```python
from build123d import *

# Parameters (mm, degrees)
F0_W     = 50.8
F0_H     = 50.8
F1_DEPTH = 6.35
F2_W     = 50.8
F2_H     = 6.35
F3_DEPTH = 6.604
F4_W     = 50.8
F4_H     = 50.8
F5_DEPTH = 6.35
F6_R     = 10.16
F6_R_2   = 8.255
F7_DEPTH = 50.8


with BuildPart() as f1:
    # F0 (on Top) → F1 (new body)
    with BuildSketch(Plane.XY):
        Rectangle(F0_W, F0_H)
    extrude(amount=F1_DEPTH)

    # F2 (on face) → F3 (join)
    with BuildSketch(Plane.XY.offset(6.35)):
        with Locations((0, 22.225)):
            Rectangle(F2_W, F2_H)
    extrude(amount=F3_DEPTH)

    # F4 (on face) → F5 (join)
    with BuildSketch(Plane.XY.offset(12.954)):
        Rectangle(F4_W, F4_H)
    extrude(amount=F5_DEPTH)

    # F6 (on face) → F7 (join)
    with BuildSketch(Plane.XY.offset(19.304)):
        Circle(F6_R)
        Circle(F6_R_2, mode=Mode.SUBTRACT)
    extrude(amount=F7_DEPTH)


solid = f1.part
```
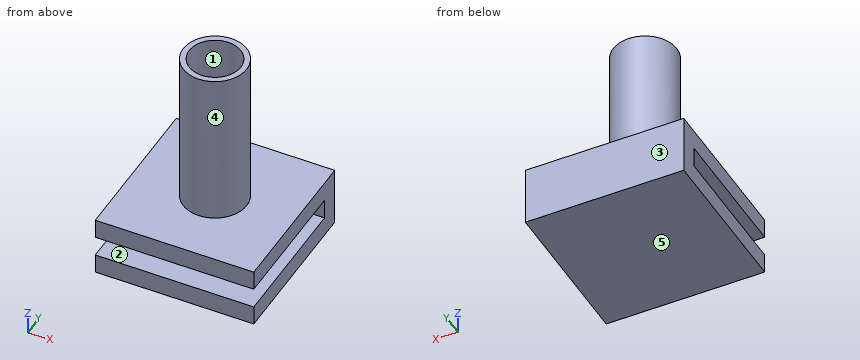
Input: part model. Units: mm. Frame: model coordinates. Face numbers are marked on the shaded views. A direction names the side the tool comes from. Coordinates: 2 decimals unless noted, no trailing zeros. Loops run counter-clockwise (first coordinate to the right, second up) from the corner with the lowest first, then second, coordinate; pieces in that order, holes last.
Q1. Line query: line 1 along Z through (x, y) = (2.5, -16); line 2 along X through (y, z) = (0.5, 19.5); line 3 along Y through (x, z) = (0, 44) (3 decimals). Output: solid intervals per line, ascending.
Results are:
line 1: z = 0 to 6.35, 12.95 to 19.3
line 2: x = -10.15 to -8.24, 8.24 to 10.15
line 3: y = -10.16 to -8.255, 8.255 to 10.16
Q2. Mould query, pull axis Y, two halves, no side actions, for the marked faces 1, 2 and 3. Classes: +Y half, -Y half, draft (parallel to the pull), parting line (faces both ways), or undercut.
Results are:
face 1: undercut
face 2: draft
face 3: +Y half
Q3. Section A-A, the plane y = 0. Return the cut outline in (x, z) (3 decimals).
Results are:
outline: (-25.4, 0) - (25.4, 0) - (25.4, 6.35) - (-25.4, 6.35) - close; (-25.4, 12.954) - (25.4, 12.954) - (25.4, 19.304) - (10.16, 19.304) - (10.16, 70.104) - (8.255, 70.104) - (8.255, 19.304) - (-8.255, 19.304) - (-8.255, 70.104) - (-10.16, 70.104) - (-10.16, 19.304) - (-25.4, 19.304) - close
Q4. Set-up query: the marked faces 4 and 5. Return all of +Z, -Z, +X, -X, +Y, -Y with unobstructed straight access to the full face (end or side cutting, diameter ignored); none if empty.
Results are:
face 4: +Z
face 5: -Z, +X, -X, +Y, -Y
Q5. Section D-D, the plane y = 15.5. Return the cut outline in (x, z).
Results are:
outline: (-25.4, 0) - (25.4, 0) - (25.4, 6.35) - (-25.4, 6.35) - close; (-25.4, 12.95) - (25.4, 12.95) - (25.4, 19.3) - (-25.4, 19.3) - close
Q6. Section C-C, the plane z = 52.5. Return the cut outline in (x, y) (3 decimals).
Results are:
outline: circle Ø20.32 at (0, 0); hole circle Ø16.51 at (0, 0)
Q7. Contact query for flat-ended pins moving along their axis: pin 1 (3.5 mm diameter, centred on x = 6.5, z = 8, fed in from -Y); pin 2 (5 mm diameter, centred on x = -11.5, z = 9.5, fed in from -Y); pin 3 (4 mm diameter, centred on y = 10.5, z = 62, fed in from +X); pin 4 (1 mm diameter, centred on x = 6.5, z = 47.5, fed in from -Y). Output: stop coordinate, or through.
Results are:
pin 1: stops at y = -25.4
pin 2: stops at y = 19.05
pin 3: stops at x = 5.57
pin 4: stops at y = -8.2
Q8. Section B-B, the plane x = -17. Return the cut outline in (y, z).
Results are:
outline: (-25.4, 0) - (25.4, 0) - (25.4, 19.3) - (-25.4, 19.3) - (-25.4, 12.95) - (19.05, 12.95) - (19.05, 6.35) - (-25.4, 6.35) - close
